Input: part model. Units: mm. Frame: model coordinates. A direction names the side the tool comes from. Coordinates: 2 decimals unless noted, no trailing zeros. Loops run counter-clockwise (first coordinate to the right, second up) from the corner with the lowest first, then second, coordinate; pieces in that order, holes last.
(1) Set-up query: faces 5 (the face through (0, 9.525, 6)), 6 (the face through (0, 0, 12.7)), 7 (the face through (0, -9.525, 6)). Return all of +Z, -Z, +X, -X, +Y, -Y with unobstructed straight access to the full face (end or side cutting, diameter ignored); none if empty.
(2) Section A-A, the plane y = 0. Give the number of separate pieces and of enclosed holes in the cut face, then the cut area to 3 significant figures.
(3) Section C-C, the plane x = -4. Return loops of the section in (y, z) (3 decimals), then the cut area to 3 significant figures.
(4) Section B-B, the plane z = 5.5. Return loops of the section in (x, y) (3 decimals).
(5) Mould query, pull axis Z, two halves, no side actions, for faces 1 (the face through (13.784, 0.079, 6.261)), 2 (the face through (-36.5, 0.2, 7.6)), 3 (the face through (-26, 0, 19.05)), 4 (the face through (0, 0, 0)). Classes: released by +Z, released by -Z, zero draft, split by the parting line, or undercut.
(6) Line query: L1, parallel to Z at x = -32.7, y = 5; L2, parallel to Y at x = -4, z = 8 (3 decimals); L3, parallel to Z at x = -18.5, y = 5.75. Output: solid intervals per line, ascending.
(7) Contact query for flat-ended pins moving along their axis: P1, Ø5.5, axis at x = 12, y = 0, coming from the -Z side; P2, Ø8, axis at y = 2, z = 10.5, coming from the -X side; P3, Ø6.5, axis at x = -6, z = 6, coming from the +Y side (3 decimals); P4, Ø2, axis at y = 8, z = 13.5, coming from the +X side. Output: stop coordinate, or through.
```python
from build123d import *

# Parameters (mm, degrees)
F0_W     = 40
F0_H     = 19.05
F1_DEPTH = 12.7
F2_W     = 25.4
F2_H     = 25.4
F2_W_2   = 19.05
F2_H_2   = 12.7
F3_DEPTH = 25.4
F5_D     = 8
F6_R     = 12.69999
F8_D     = 3.571875


# Not quite as in the source:
# - a fillet or chamfer is up to 0.001 mm smaller than in the source, because OpenCascade refuses the exact size


with BuildPart() as f1:
    # F0 (on Top) → F1 (new body)
    with BuildSketch(Plane.XY):
        Rectangle(F0_W, F0_H)
    extrude(amount=F1_DEPTH)

    # F2 (on face) → F3 (join)
    with BuildSketch(Plane(origin=(-20, 0, 0), x_dir=(0, -1, 0), z_dir=(-1, 0, 0))):
        with Locations((0, 6.35)):
            Rectangle(F2_W, F2_H)
        with Locations((0, 6.35)):
            Rectangle(F2_W_2, F2_H_2, mode=Mode.SUBTRACT)
        with Locations((0, 6.35)):
            Rectangle(F2_W_2, F2_H_2)
    extrude(amount=F3_DEPTH)

    # F5 (through all)
    with Locations(Plane.XZ.offset(12.7)):
        with Locations((-32.7, 6.35)):
            Hole(F5_D / 2)

    # F6 (radius 12.7 in the source; OpenCascade refuses exactly that, so slightly less here)
    f6_edges = [f1.edges().sort_by_distance(p)[0] for p in [
        (-45.4, 0, 19.05),
        (-45.4, 0, -6.35),
    ]]
    fillet(f6_edges, radius=F6_R)

    # F8 (through all)
    with Locations(Plane.XY.offset(12.7)):
        with Locations((12, 0), (-4, 0)):
            Hole(F8_D / 2)


solid = f1.part
```
Report:
1. face 5: +Z, -Z, +X, +Y
1. face 6: +Z, +X, +Y, -Y
1. face 7: +Z, -Z, +X, -Y
2. separate pieces: 3
2. enclosed holes: 1
2. area: 943 mm2
3. outline: (-9.525, 0) - (-1.786, 0) - (-1.786, 12.7) - (-9.525, 12.7) - close; (1.786, 0) - (9.525, 0) - (9.525, 12.7) - (1.786, 12.7) - close
3. area: 197 mm2
4. outline: (-45.372, -12.7) - (-36.609, -12.7) - (-36.609, 12.7) - (-45.372, 12.7) - close; (-28.791, -12.7) - (-20, -12.7) - (-20, -9.525) - (20, -9.525) - (20, 9.525) - (-20, 9.525) - (-20, 12.7) - (-28.791, 12.7) - close; hole circle Ø3.572 at (-4, 0); hole circle Ø3.572 at (12, 0)
5. face 1: zero draft
5. face 2: undercut
5. face 3: released by +Z
5. face 4: released by -Z
6. L1: z = -6.35 to 2.35, 10.35 to 19.05
6. L2: y = -9.525 to -1.786, 1.786 to 9.525
6. L3: z = 0 to 12.7
7. P1: stops at z = 0
7. P2: stops at x = -45.4
7. P3: stops at y = 9.525
7. P4: stops at x = 20
